Geometry: final body of the model. Coordinates: model frame, mm. Face numbers are marked on the shaded views. A direction names the side the tool comes from. Give positions to 0.01 mm unless a question says otherwise; leave off trailing zeros. Write each loop counter-clockwise with the first axis right and the second up, starting at its lowest first coordinate (ties: lowest second). Pieces come first, ordered by that corner, then holes. Notation, with made-up numbers: M 66,35.25 L 116,35.25 A21 cw 116,59.25 Z; hole C 88,4.5 d2. An arc over 180 degrees is marked long. Use one line per item in the form item = value. Start each with the question number.
Item 1: Section query D-D on z = 22. Return loops of the section in (x, y).
Item 2: Access query for the marked faces 1 and 2. Directions: +Z, -Z, +X, -X, +Y, -Y. A direction counts if a zero-diameter tool reaches every point of the face in a straight line with its end or side. Return the directions, or none.
Item 3: Section query C-C on x = 56. Return loops of the section in (y, z), then the cut area to 3 significant figures.
Item 4: Pull-direction query (Y, two-part tool) for the marked faces 3, 4, 5 and 6; classes: released by +Y, released by -Y, zero draft, split by the parting line, or undercut.
Item 5: Section query B-B on z = 14. Return loops of the section in (x, y), then the cut area to 3 significant figures.
Item 6: Section query A-A on y = 27. Return loops of the section in (x, z) (3 decimals), then the cut area to 3 significant figures.
Item 7: Material intervals for line 1 along X through (y, z) = (20.5, 26.5); line 2 along Y through (x, z) = (22, 19.5); line 3 along Y through (x, z) = (36, 21.5), sorted ascending. Write a range as from..to.
Item 8: Contact query for flat-ended pins moving along their axis: P1, Ø16, axis at y = 20.5, z = 22, coming from the +X side; P2, Ø5, axis at y = 24, z = 16, coming from the -X side; P3, Ø10, axis at y = 14.5, z = 17, coming from the +X side. Output: stop coordinate, or through.
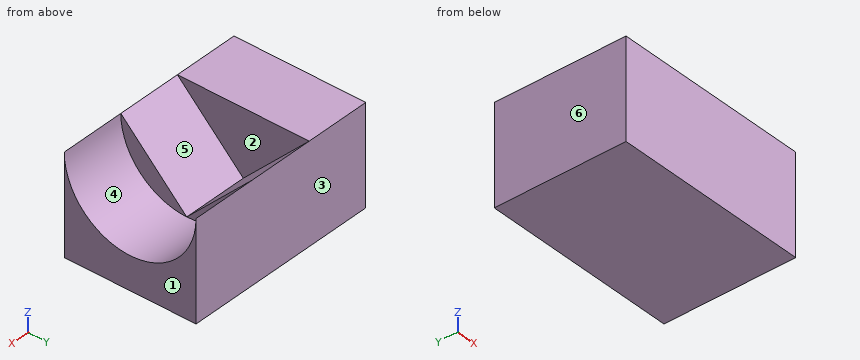
from build123d import *

# Parameters (mm, degrees)
F0_W     = 60
F0_H     = 40
F1_DEPTH = 30
F3_DEPTH = 20
F5_DEPTH = 20


with BuildPart() as f1:
    # F0 (on Top) → F1 (new body)
    with BuildSketch(Plane.XY):
        with Locations((30, 20)):
            Rectangle(F0_W, F0_H)
    extrude(amount=F1_DEPTH)

    # F2 (on face) → F3 (cut)
    with BuildSketch(Plane.YZ.offset(60)):
        with BuildLine():
            Line((40, 30), (0, 30))
            ThreePointArc((0, 30), (20, 10), (40, 30))
        make_face()
    extrude(amount=-F3_DEPTH, mode=Mode.SUBTRACT)

    # F4 (on face) → F5 (cut)
    with BuildSketch(Plane.YZ.offset(40)):
        Polygon((40, 30), (0, 30), (20, 10), align=None)
    extrude(amount=-F5_DEPTH, mode=Mode.SUBTRACT)


solid = f1.part
Answer sheet:
q1.outline = M 0,0 L 60,0 L 60,1.67 L 40,1.67 L 40,8 L 20,8 L 20,32 L 40,32 L 40,38.33 L 60,38.33 L 60,40 L 0,40 Z
q2.face_1 = +Z, -Z, +X, +Y, -Y
q2.face_2 = +Z, +X
q3.outline = M 0,0 L 40,0 L 40,30 A20 cw 0,30 Z
q3.area = 572 mm2
q4.face_3 = released by +Y
q4.face_4 = undercut
q4.face_5 = undercut
q4.face_6 = zero draft
q5.outline = M 0,0 L 60,0 L 60,8 L 40,8 L 40,16 L 20,16 L 20,24 L 40,24 L 40,32 L 60,32 L 60,40 L 0,40 Z
q5.area = 1,760 mm2
q6.outline = M 0,0 L 60,0 L 60,11.265 L 40,11.265 L 40,17 L 20,17 L 20,30 L 0,30 Z
q6.area = 1,170 mm2
q7.line_1 = 0..20
q7.line_2 = 0..10.5, 29.5..40
q7.line_3 = 0..8.5, 31.5..40
q8.P1 = 20
q8.P2 = 0
q8.P3 = 40
